from build123d import *

# Parameters (mm, degrees)
F0_W     = 330.2
F0_H     = 63.5
F1_DEPTH = 19.05
F3_DEPTH = 63.501
F5_DEPTH = 19.051
F7_DEPTH = 63.5


with BuildPart() as f1:
    # F0 (on Right) → F1 (new body)
    with BuildSketch(Plane.YZ):
        with Locations((-165.1, 31.75)):
            Rectangle(F0_W, F0_H)
    extrude(amount=F1_DEPTH)

    # F2 (on face) → F3 (cut, through all)
    with BuildSketch(Plane.XY.offset(63.5)):
        Polygon((0, -1.666659), (19.05, 0), (0, 0), align=None)
    extrude(amount=-F3_DEPTH, mode=Mode.SUBTRACT)

    # F4 (on face) → F5 (cut, through all)
    with BuildSketch(Plane.YZ.offset(19.05)):
        Polygon((-324.64447, 63.5), (-330.2, 63.5), (-330.2, 0), align=None)
    extrude(amount=-F5_DEPTH, mode=Mode.SUBTRACT)

    # F6 (on face) → F7 (join)
    with BuildSketch(Plane.XY.offset(63.5)):
        Polygon((19.05, -324.64447), (0, -324.64447), (0, -326.311129), align=None)
    extrude(amount=-F7_DEPTH)


solid = f1.part
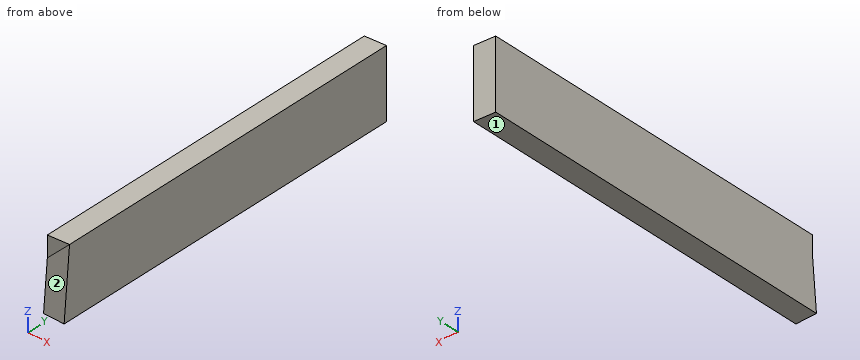
For this review, take the finished solid that the model builds, in its own axes (mm). Face numbers are marked on the shaded views. A direction names the side the tool comes from. Give positions to 0.01 mm unless a question says otherwise; leave off trailing zeros. Answer as a JSON object with one key per item and string values. Group by question number.
Item 1: Wall thickness on line 1 along Y through (x, z) = (5.25, 30); line 2 along Y through (x, z) = (9.75, 10): over which ranges is each line inside the solid? List them lowest first.
Item 2: Clearance check with flat-ended pins moving along their axes: pin 1 Ø2 at (x, y) = (3, -97) entering from -Z; pin 2 Ø8 at (x, z) = (15, 44) entering from -Y; pin 3 Ø2 at (x, z) = (7.5, 8) entering from -Y; pin 4 Ø8 at (x, z) = (4, 8.5) entering from +Y. State where each tip first meets the part, or that it passes through.
Item 3: Machinability: for the marked faces 1 and 2, which of the approach directions +Z, -Z, +X, -X, +Y, -Y give a long, thin tool a straight path to every point of the face, cutting with its end or side? Answer none if there is none.
Reported:
{
 "1": {"line 1": "-327.58 to -1.21", "line 2": "-329.33 to -0.81"},
 "2": {"pin 1": "z = 0", "pin 2": "y = -326.7", "pin 3": "y = -329.59", "pin 4": "y = -0.97"},
 "3": {"face 1": "-Z, +X, -X, +Y, -Y", "face 2": "+Z, +X, -Y"}
}
